CAD build for the part. Positions are in the model's coordinates, mm. Round coordinates to 2 decimals unless told otherwise and drop trailing zeros. Loops run counter-clockwise (first coordinate to the right, second up) from the corner with the lowest first, then second, coordinate; pieces in that order, holes last. Notation, with made-up numbers: M -40,22.25 L 19,22.25 A11 cw 19,29.25 Z; hole C 69.25,77 d7. An arc over 180 degrees is marked long. Use one line per item in the form item = value.
from build123d import *

# Parameters (mm, degrees)
BOSS_EXTRU_1_DEPTH      = 5
ESQUISSE2_W             = 10
ESQUISSE2_H             = 5
ESQUISSE2_W_2           = 5
ESQUISSE2_H_2           = 10
ENL_V_MAT_EXTRU_2_DEPTH = 600.103496902


with BuildPart() as part:
    # Esquisse1 → Boss.-Extru.1 (new body)
    with BuildSketch(Plane.XY):
        Polygon((400, 20), (400, 330), (500, 330), (500, 0), (400, 0), (0, 0), (0, 20), align=None)
    extrude(amount=BOSS_EXTRU_1_DEPTH)

    # Esquisse2 → Enlèv. mat.-Extru.2 (cut, through all)
    with BuildSketch(Plane.XY.offset(5)):
        with Locations((25, 2.5)):
            Rectangle(ESQUISSE2_W, ESQUISSE2_H)
        with Locations((5, 2.5)):
            Rectangle(ESQUISSE2_W, ESQUISSE2_H)
        with Locations((45, 2.5)):
            Rectangle(ESQUISSE2_W, ESQUISSE2_H)
        with Locations((65, 2.5)):
            Rectangle(ESQUISSE2_W, ESQUISSE2_H)
        with Locations((85, 2.5)):
            Rectangle(ESQUISSE2_W, ESQUISSE2_H)
        with Locations((105, 2.5)):
            Rectangle(ESQUISSE2_W, ESQUISSE2_H)
        with Locations((125, 2.5)):
            Rectangle(ESQUISSE2_W, ESQUISSE2_H)
        with Locations((145, 2.5)):
            Rectangle(ESQUISSE2_W, ESQUISSE2_H)
        with Locations((165, 2.5)):
            Rectangle(ESQUISSE2_W, ESQUISSE2_H)
        with Locations((185, 2.5)):
            Rectangle(ESQUISSE2_W, ESQUISSE2_H)
        with Locations((205, 2.5)):
            Rectangle(ESQUISSE2_W, ESQUISSE2_H)
        with Locations((225, 2.5)):
            Rectangle(ESQUISSE2_W, ESQUISSE2_H)
        with Locations((245, 2.5)):
            Rectangle(ESQUISSE2_W, ESQUISSE2_H)
        with Locations((265, 2.5)):
            Rectangle(ESQUISSE2_W, ESQUISSE2_H)
        with Locations((285, 2.5)):
            Rectangle(ESQUISSE2_W, ESQUISSE2_H)
        with Locations((305, 2.5)):
            Rectangle(ESQUISSE2_W, ESQUISSE2_H)
        with Locations((325, 2.5)):
            Rectangle(ESQUISSE2_W, ESQUISSE2_H)
        with Locations((345, 2.5)):
            Rectangle(ESQUISSE2_W, ESQUISSE2_H)
        with Locations((365, 2.5)):
            Rectangle(ESQUISSE2_W, ESQUISSE2_H)
        with Locations((385, 2.5)):
            Rectangle(ESQUISSE2_W, ESQUISSE2_H)
        with Locations((405, 2.5)):
            Rectangle(ESQUISSE2_W, ESQUISSE2_H)
        with Locations((425, 2.5)):
            Rectangle(ESQUISSE2_W, ESQUISSE2_H)
        with Locations((445, 2.5)):
            Rectangle(ESQUISSE2_W, ESQUISSE2_H)
        with Locations((465, 2.5)):
            Rectangle(ESQUISSE2_W, ESQUISSE2_H)
        Polygon((480, 0), (480, 5), (490, 5), (500, 5), (500, 0), (490, 0), align=None)
        with Locations((497.5, 315)):
            Rectangle(ESQUISSE2_W_2, ESQUISSE2_H_2)
        with Locations((497.5, 295)):
            Rectangle(ESQUISSE2_W_2, ESQUISSE2_H_2)
        with Locations((497.5, 275)):
            Rectangle(ESQUISSE2_W_2, ESQUISSE2_H_2)
        with Locations((497.5, 255)):
            Rectangle(ESQUISSE2_W_2, ESQUISSE2_H_2)
        with Locations((497.5, 235)):
            Rectangle(ESQUISSE2_W_2, ESQUISSE2_H_2)
        with Locations((497.5, 215)):
            Rectangle(ESQUISSE2_W_2, ESQUISSE2_H_2)
        with Locations((497.5, 195)):
            Rectangle(ESQUISSE2_W_2, ESQUISSE2_H_2)
        with Locations((497.5, 175)):
            Rectangle(ESQUISSE2_W_2, ESQUISSE2_H_2)
        with Locations((497.5, 155)):
            Rectangle(ESQUISSE2_W_2, ESQUISSE2_H_2)
        with Locations((497.5, 135)):
            Rectangle(ESQUISSE2_W_2, ESQUISSE2_H_2)
        with Locations((497.5, 115)):
            Rectangle(ESQUISSE2_W_2, ESQUISSE2_H_2)
        with Locations((497.5, 95)):
            Rectangle(ESQUISSE2_W_2, ESQUISSE2_H_2)
        with Locations((497.5, 75)):
            Rectangle(ESQUISSE2_W_2, ESQUISSE2_H_2)
        with Locations((497.5, 55)):
            Rectangle(ESQUISSE2_W_2, ESQUISSE2_H_2)
    extrude(amount=-ENL_V_MAT_EXTRU_2_DEPTH, mode=Mode.SUBTRACT)


solid = part.part
1. Cut at B-B on y = 29.5. Write the cut outline in (x, z), and give its area (3 significant figures).
Completed:
outline = M 400,0 L 500,0 L 500,5 L 400,5 Z
area = 500 mm2
2. Cut at A-A on x = 175. Write the cut outline in (y, z), and give its area (3 significant figures).
Completed:
outline = M 0,0 L 20,0 L 20,5 L 0,5 Z
area = 100 mm2
3. Probe line 1 along X through (y, z) = (117, 3.15); line 2 along Y through (x, z) = (147, 0.9); line 3 along Y through (x, z) = (199.5, 3.7). List the from-to ranges inside material, lowest first. Write a range as from..to.
Completed:
line_1 = 400..495
line_2 = 5..20
line_3 = 0..20
4. Drop flat-ended pins along their axis: P1, Ø1.5, axis at y = 3.5, z = 2.5, coming from the -X side; P2, Ø1.5, axis at y = 314, z = 3, coming from the +X side; P3, Ø2, axis at y = 148.5, z = 1.5, coming from the -X side. Give the stop position or say it passes through.
Completed:
P1 = 10
P2 = 495
P3 = 400
